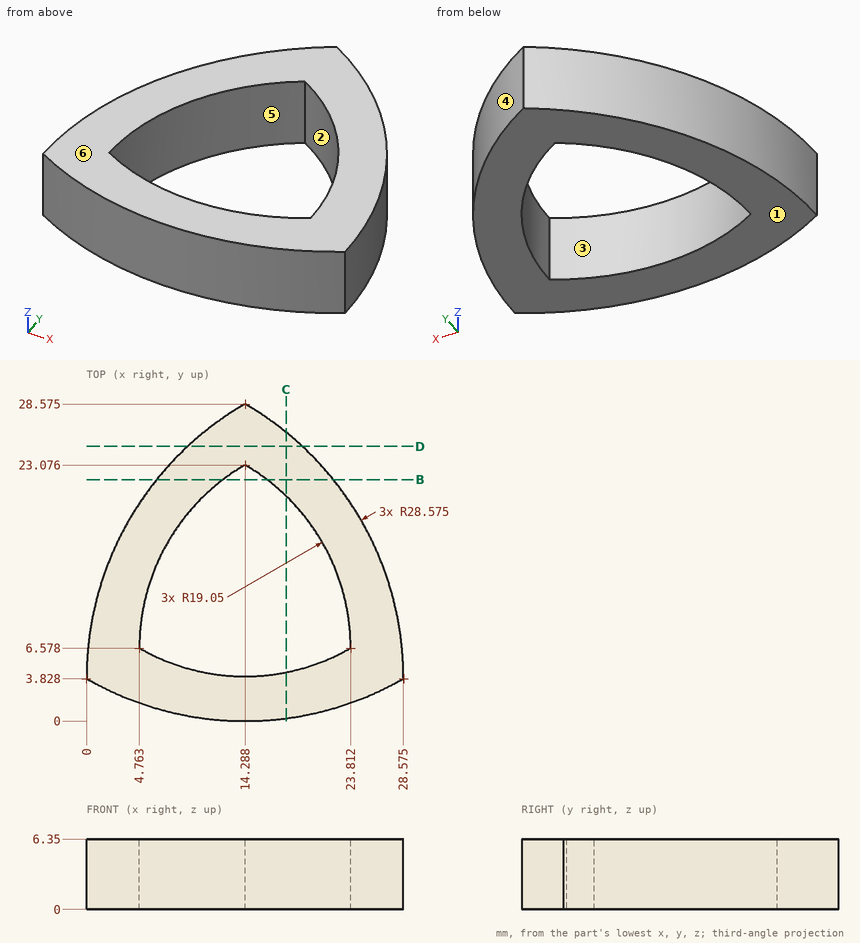
Geometry: see drawing. Coordinates: mm, zero at the bounding-box minimum. A direction names the side the tool comes from. Coordinates: 2 decimals unless noted, no trailing zeros. Order: outer loops, then holes, each group sorted by start corner. A loop starts at its lowest first (then second) coordinate and runs counter-clockwise, first axis right, second up. Notation, with made-up numbers: M -20.75,-6.5 L 18.25,-6.5 A18 ccw 18.25,7.5 Z; hole C 74,-23 d10. An arc over 180 degrees is marked long. Answer in a Markdown table with one row per item. Add a question column.
Q1. Line query: L1, parallel to X at y = 14.75, z = 0.75 (1 decimal); L2, parallel to X at y = 16.75, z = 3.5 (1 decimal); L3, parallel to Y at x = 17.25, z = 4.75 (1 decimal). Output: solid intervals per line, ascending.
Q2. Section query D-D on y = 24.75. Return the cut outline in (x, z).
Q3. Mould query, pull axis Y, two halves, no side actions, for the marked faces 1, 2, 3 and 4. Classes: released by +Y, released by -Y, zero draft, split by the parting line, or undercut.
Q4. Contact query for flat-ended pins moving along their axis: P1, Ø1, axis at y = 22.5, z = 5.5, coming from the +X side; P2, Ø1.5, axis at y = 5, z = 5.5, coming from the +X side; P3, Ø3, axis at x = 11.5, z = 1, coming from the +Y side (1 decimal). Output: stop coordinate, or through.
Q5. Section query B-B on y = 21.75. Return the cut outline in (x, z).
Q6. Reachability of the marked faces 5 and 6 from +Z, -Z, +X, -X, +Y, -Y: full face, straight path, thin tool, end or side. Return the list, or none.
Q7. Section query C-C on x = 18. Return the cut outline in (y, z).
Completed:
| question | item | result |
|---|---|---|
| 1 | L1 | x = 2.2 to 6.6, 22 to 26.4 |
| 1 | L2 | x = 3.1 to 7.7, 20.9 to 25.5 |
| 1 | L3 | y = 0.2 to 4.3, 21 to 26.6 |
| 2 | outline | M 9.11,0 L 19.46,0 L 19.46,6.35 L 9.11,6.35 Z |
| 3 | face 1 | zero draft |
| 3 | face 2 | undercut |
| 3 | face 3 | undercut |
| 3 | face 4 | released by +Y |
| 4 | P1 | stops at x = 22.05 |
| 4 | P2 | stops at x = 28.57 |
| 4 | P3 | stops at y = 27.8 |
| 5 | outline | M 6.32,0 L 12.29,0 L 12.29,6.35 L 6.32,6.35 Z; M 16.28,0 L 22.26,0 L 22.26,6.35 L 16.28,6.35 Z |
| 6 | face 5 | +Z, -Z |
| 6 | face 6 | +Z, +X, -X, +Y, -Y |
| 7 | outline | M 0.24,0 L 4.39,0 L 4.39,6.35 L 0.24,6.35 Z; M 20.28,0 L 26.02,0 L 26.02,6.35 L 20.28,6.35 Z |
